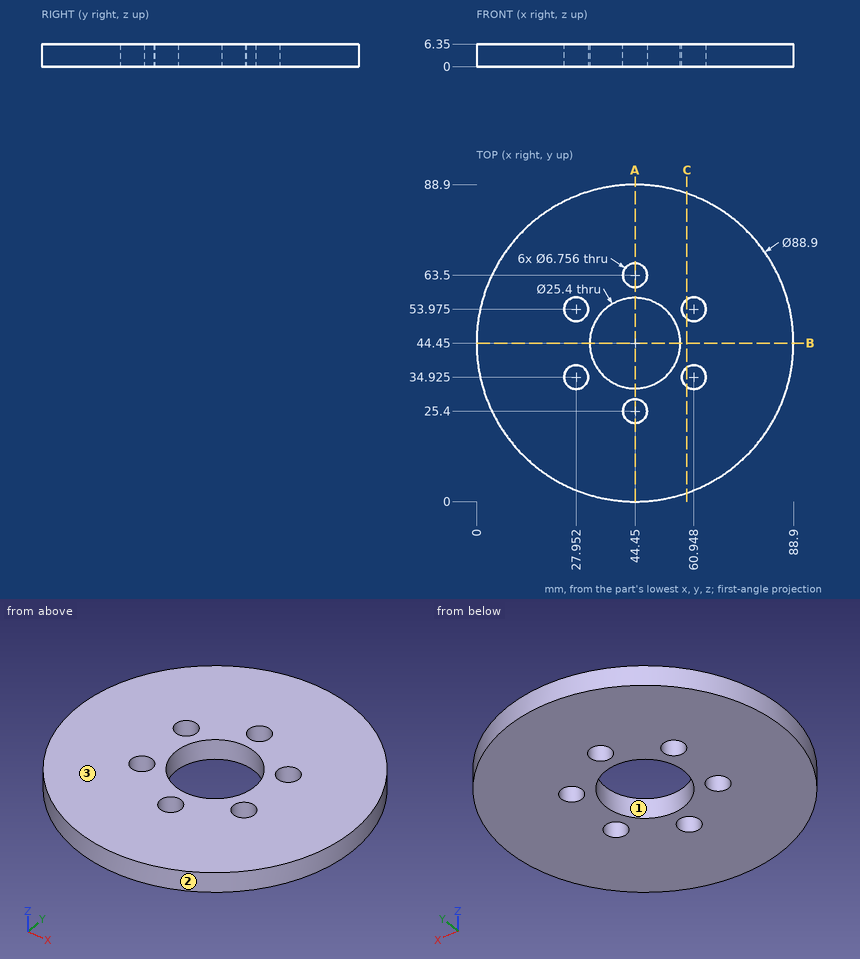
Source: three-view drawing plus pictorial views. Frame: mm from the lowest corner of the part. Give positions to 0.01 mm unless a question says otherwise; leave off trailing zeros. Order: outer loops, then holes, each group sorted by start corner. A loop starts at its lowest first (then second) coordinate and runs counter-clockwise, first axis right, second up. Notation, with made-up numbers: M -36,-33.75 L -23,-33.75 A26 ccw -23,-11.75 Z; hole C -19.75,30.5 d11. An arc over 180 degrees is marked long. One line per question, with ' | ' between items.
1) Contact query for flat-ended pins moving along their axis: P1, Ø1.5, axis at y = 74.5, z = 2, coming from the -X side (1 decimal); P2, Ø1, axis at x = 29.5, z = 1, coming from the +Y side (1 decimal); P3, Ø6, axis at x = 27.95, y = 34.93, coming from the +Z side (1 decimal). Output: stop coordinate, or through.
Filled in:
P1: stops at x = 11 | P2: stops at y = 86.5 | P3: passes through
2) Section A-A on x = 44.45. Output: boundary loops of the cut face in (y, z).
Filled in:
outline: M 0,0 L 22.02,0 L 22.02,6.35 L 0,6.35 Z; M 28.78,0 L 31.75,0 L 31.75,6.35 L 28.78,6.35 Z; M 57.15,0 L 60.12,0 L 60.12,6.35 L 57.15,6.35 Z; M 66.88,0 L 88.9,0 L 88.9,6.35 L 66.88,6.35 Z
3) Section C-C on x = 59. State how many separate pieces and enclosed holes the cut face has, and give its area (3 significant figures).
Filled in:
separate pieces: 3 | enclosed holes: 0 | area: 463 mm2
4) Draft query along X for the marked faces 1, 2 and 3. Return one class per face: pulls with the +X half, pulls with the -X half, needs draft (parallel to the pull), parting line crosses it, or undercut.
Filled in:
face 1: undercut | face 2: parting line crosses it | face 3: needs draft
5) Ray query, L1, parallel to Y at x = 44.45, z = 3.5; L2, parallel to X at y = 37.5, z = 3 (1 decimal); L3, parallel to Y at x = 25.5, z = 6. Return the intervals inside material, ascending.
Filled in:
L1: y = 0 to 22.02, 28.78 to 31.75, 57.15 to 60.12, 66.88 to 88.9 | L2: x = 0.5 to 25.8, 30.1 to 33.8, 55.1 to 58.8, 63.1 to 88.4 | L3: y = 4.24 to 32.6, 37.25 to 51.65, 56.3 to 84.66
6) Section B-B on y = 44.45. Output: boundary loops of the cut face in (x, z), and give its area (3 significant figures).
Filled in:
outline: M 0,0 L 31.75,0 L 31.75,6.35 L 0,6.35 Z; M 57.15,0 L 88.9,0 L 88.9,6.35 L 57.15,6.35 Z | area: 403 mm2
